Verification items for the finished model (mm, model axes). Round coordinates to 2 decimals unless told otherwise and drop trailing zeros. Order: outer loops, then holes, each group sorted by start corner. A loop starts at its lowest first (then second) coordinate and runs counter-clockwise, first axis right, second up. Notation, with made-up numbers: (-15.75, 48) -> (-0.75, 48) arc R21 cw to (-0.75, 52) -> close; hole circle Ø4 at (-31, -23.5). An arc over 180 degrees is marked (long way). Put each result on its own line as item: value.
from build123d import *

# Parameters (mm, degrees)
SKETCH1_W            = 123.075797847
SKETCH1_H            = 17.9
SKETCH1_R            = 2
SKETCH1_R_2          = 2.54
BASE_FLANGE1_DEPTH   = 3.175
FILLET1_R            = 2.54
M8_CLEARANCE_HOLE1_D = 9
M6_CLEARANCE_HOLE1_D = 6.6
SKETCH10_R           = 1
CUT_EXTRUDE1_DEPTH   = 79.592687586
M3_CLEARANCE_HOLE2_D = 3.4


# Sheet-metal steps are written as plain solids
with BuildPart() as part:
    # Sketch1 → Base-Flange1 (new body)
    with BuildSketch(Plane.XY):
        with Locations((13.466115103, 14.312153748)):
            Rectangle(SKETCH1_W, SKETCH1_H)
        with Locations((-39.121783821, 14.312153748)):
            Circle(SKETCH1_R, mode=Mode.SUBTRACT)
        with Locations((68.323814026, 15.635739427)):
            Circle(SKETCH1_R_2, mode=Mode.SUBTRACT)
    extrude(amount=-BASE_FLANGE1_DEPTH)

    # Fillet1
    fillet1_edges = [part.edges().sort_by_distance(p)[0] for p in [
        (-48.071783821, 23.262153748, -1.5875),
        (75.004014026, 23.262153748, -1.5875),
        (75.004014026, 5.362153748, -1.5875),
        (-48.071783821, 5.362153748, -1.5875),
    ]]
    fillet(fillet1_edges, radius=FILLET1_R)

    # M8 Clearance Hole1 (through all)
    with Locations(Plane.XY):
        with Locations((-39.121783821, 14.312153748)):
            Hole(M8_CLEARANCE_HOLE1_D / 2)

    # M6 Clearance Hole1 (through all)
    with Locations(Plane.XY):
        with Locations((68.323814026, 15.635739427)):
            Hole(M6_CLEARANCE_HOLE1_D / 2)

    # Sketch10 → Cut-Extrude1 (cut, through all)
    with BuildSketch(Plane.XY):
        with Locations((13.466115103, 14.312153748)):
            Circle(SKETCH10_R)
    extrude(amount=-CUT_EXTRUDE1_DEPTH, mode=Mode.SUBTRACT)

    # M3 Clearance Hole2 (through all)
    with Locations(Plane.XY):
        with Locations((13.466115103, 14.312153748)):
            Hole(M3_CLEARANCE_HOLE2_D / 2)


solid = part.part
Item 1: Gauge pin test, flat end, axial feed: pin 1 Ø2 at (x, y) = (13.47, 14.31) entering from -Z. Record the tip position at first contact, or that the pin passes through.
Check sheet entries:
pin 1: passes through
Item 2: Section check B-B on z = -1.7. Record the boundary of the cut face in (x, y), then the cut area to 3 significant figures.
Check sheet entries:
outline: (-48.07, 7.9) arc R2.54 ccw to (-45.53, 5.36) -> (72.46, 5.36) arc R2.54 ccw to (75, 7.9) -> (75, 20.72) arc R2.54 ccw to (72.46, 23.26) -> (-45.53, 23.26) arc R2.54 ccw to (-48.07, 20.72) -> close; hole circle Ø9 at (-39.12, 14.31); hole circle Ø3.4 at (13.47, 14.31); hole circle Ø6.6 at (68.32, 15.64)
area: 2,090 mm^2
Item 3: Release check for a two-part mould opening along Y. For faces 1 (the cylindrical face through (74.24, 22.54, -1.61)), 2 (the flat face through (13, 5.362, -2)), 3 (the cylindrical face through (-43.414, 15.664, -1.61)), 4 (the cylindrical face through (65.275, 14.372, -1.61)) record: +Y half, -Y half, draft (parallel to the pull), parting line (faces both ways), or undercut.
Check sheet entries:
face 1: +Y half
face 2: -Y half
face 3: undercut
face 4: undercut
Item 4: Section check A-A on x = 13. Record the boundary of the cut face in (y, z) (3 decimals), then the cut area to 3 significant figures.
Check sheet entries:
outline: (5.362, -3.175) -> (12.677, -3.175) -> (12.677, 0) -> (5.362, 0) -> close; (15.947, -3.175) -> (23.262, -3.175) -> (23.262, 0) -> (15.947, 0) -> close
area: 46.5 mm^2
Item 5: Material ranges on L1, parallel to X at y = 17, z = -2.6; L2, parallel to X at y = 18, z = -0.8; L3, parallel to X at y = 15.25, z = -1.5, recorded low to high. Write a range as [from, to].
Check sheet entries:
L1: x = [-48.07, -42.73], [-35.51, 65.32], [71.33, 75]
L2: x = [-48.07, -41.7], [-36.54, 66.02], [70.63, 75]
L3: x = [-48.07, -43.52], [-34.72, 12.05], [14.88, 65.05], [71.6, 75]
